Read the model definition and answer for the solid it produces. Units are mm, in the model's axes. Face numbers are marked on the shaded views. A direction names the side the tool comes from. Give positions to 0.01 mm unless a question says otherwise; leave off trailing zeros. Write each loop counter-clockwise with the first axis right and the second up, starting at its lowest first coordinate (ties: lowest second). Pieces come first, ordered by that corner, then holes. Notation, with made-up numbers: (9.5, 24) - (34.5, 24) arc R20 cw to (34.5, 33) - close; hole circle Ø7 at (88, 10). An arc over 180 degrees is marked (long way). Answer as a JSON object with one key per item and string values. Group by question number.
```python
from build123d import *

# Parameters (mm, degrees)
CHAMFER1_SIZE = 0.127


with BuildPart() as part:
    # Sketch1 → Revolve1 (revolve)
    with BuildSketch(Plane.XY):
        Polygon((0, 1.8542), (0, 2.3622), (2.032, 2.3622), (2.032, 1.397), (5.334, 1.397), (5.334, 0), (1.905, 0), (1.524, 0.634090483), (1.524, 1.8542), align=None)
    revolve(axis=Axis((0, 0, 0), (1, 0, 0)))

    # Chamfer1
    chamfer1_edges = [part.edges().sort_by_distance(p)[0] for p in [
        (2.032, -2.3622, 0),
        (5.334, -1.397, 0),
    ]]
    chamfer(chamfer1_edges, length=CHAMFER1_SIZE)


solid = part.part
```
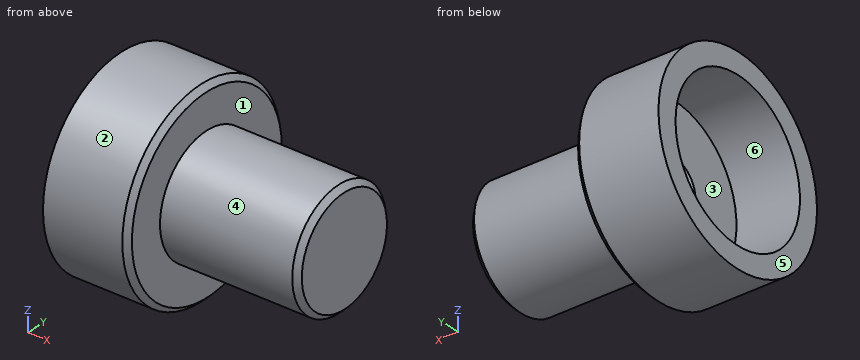
1) Find the intervals of material crossed by line 1 (Z direction, x = 0.4, y = 0); line 2 (X direction, y = 0.4, z = 2); line 3 (Y direction, x = 0.75, z = -1.15), in increasing order. Write a range as [from, to].
2) For a pull along Y with two mould halves and no side action, classify the marked faces 1, 2 and 3 as released by +Y, released by -Y, zero draft, split by the parting line, or undercut.
3) Which of the six approach directions +Z, -Z, +X, -X, +Y, -Y give full straight-line access (tool end or side, diameter ignored) to the marked faces 4, 5 and 6?
4) A flat-ended cylindrical pin translates along its axis: pin 1 Ø2 at (x, z) = (1, 1.5) entering from -Y. Find the tip coordinate at first contact, or state that the pin passes through.
5) Find section A-A, the plane x = 4.75. Write down the section's boundary in (y, z), and give its area (3 significant figures).
Values follow:
{
 "1": {"line 1": "z = [-2.36, -1.85], [1.85, 2.36]", "line 2": "x = [0, 2.03]", "line 3": "y = [-2.06, -1.45], [1.45, 2.06]"},
 "2": {"face 1": "zero draft", "face 2": "split by the parting line", "face 3": "undercut"},
 "3": {"face 4": "+X", "face 5": "+Z, -Z, -X, +Y, -Y", "face 6": "-X"},
 "4": {"pin 1": "stops at y = -2.31"},
 "5": {"outline": "circle Ø2.79 at (0, 0)", "area": "6.13 mm2"}
}
